```python
from build123d import *

# Parameters (mm, degrees)
F1_DEPTH = 72
F3_DEPTH = 30.001
F5_W     = 50
F5_H     = 6
F6_DEPTH = 72
F4_R     = 12
F7_DEPTH = 133.001
F8_DEPTH = 12.001


with BuildPart() as f1:
    # F0 (on Front) → F1 (new body)
    with BuildSketch(Plane.XZ):
        Polygon((-45.791163, 76.894684), (-81.791163, 76.894684), (-81.791163, 48.164527), (-69.791163, 48.164527), (-69.791163, 16.894684), (-81.791163, 16.894684), (-81.791163, -13.105316), (-9.791163, -13.105316), (63.208837, -13.105316), (63.208837, 16.894684), (-45.791163, 16.894684), align=None)
    extrude(amount=F1_DEPTH)

    # F2 (on face) → F3 (cut, through all)
    with BuildSketch(Plane.XY.offset(16.894684)):
        with BuildLine():
            Line((63.208837, -24), (13.208837, -24))
            ThreePointArc((13.208837, -24), (1.208837, -36), (13.208837, -48))
            Line((13.208837, -48), (63.208837, -48))
            Line((63.208837, -48), (63.208837, -24))
        make_face()
    extrude(amount=-F3_DEPTH, mode=Mode.SUBTRACT)

    # F5 (on face) → F6 (cut)
    with BuildSketch(Plane(origin=(-81.791163, 0, 0), x_dir=(0, -1, 0), z_dir=(-1, 0, 0))):
        with Locations((47, -10.105316)):
            Rectangle(F5_W, F5_H)
    extrude(amount=-F6_DEPTH, mode=Mode.SUBTRACT)

    # F4 (on face) → F7 (cut, through all)
    with BuildSketch(Plane(origin=(-69.791163, 0, 0), x_dir=(0, -1, 0), z_dir=(-1, 0, 0))):
        with Locations((36, 32.529606)):
            Circle(F4_R)
    extrude(amount=-F7_DEPTH, mode=Mode.SUBTRACT)

    # F4 (on face) → F8 (cut, through all)
    with BuildSketch(Plane(origin=(-69.791163, 0, 0), x_dir=(0, -1, 0), z_dir=(-1, 0, 0))):
        with Locations((36, 32.529606)):
            Circle(F4_R)
        with BuildLine():
            Line((61.603696, 16.894684), (10.396304, 16.894684))
            ThreePointArc((10.396304, 16.894684), (36, 2.529606), (61.603696, 16.894684))
        make_face()
        with BuildLine():
            Line((10.396304, 48.164527), (61.603696, 48.164527))
            ThreePointArc((61.603696, 48.164527), (36, 62.529606), (10.396304, 48.164527))
        make_face()
    extrude(amount=F8_DEPTH, mode=Mode.SUBTRACT)


solid = f1.part
```
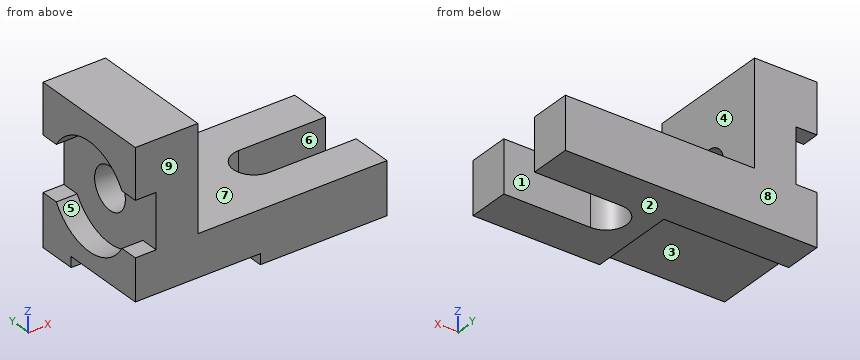
Part model, mm, in its own coordinate system. Face numbers are marked on the shaded views. A direction names the side the tool comes from. Round coordinates to 2 decimals unless told otherwise and drop trailing zeros. Order: outer loops, then holes, each group sorted by start corner. A loop starts at its lowest first (then second) coordinate and runs counter-clockwise, first axis right, second up. Notation, with made-up numbers: M 27,40.25 L 65,40.25 A30 cw 65,71.25 Z; hole C -11.5,-3 d4. An arc over 180 degrees is marked long. Put each result on its own line as item: value. Start each with the question number.
1. Slice it at D-D on y = -6.5. List the corners of the cut face in (x, z), then the cut area to 3 significant figures.
2. Drop flat-ended pins along their axis: pin 1 (3 mm diameter, centred on x = 6.5, z = -1.5, fed in from +Y); pin 2 (3 mm diameter, centred on x = -22, y = -42.5, fed in from -Z); pin 3 (21.5 mm diameter, centred on x = -3, y = -47, fed in from +Z); pin 4 (1.8 mm diameter, centred on x = -55.5, z = -11, fed in from -Y). Give the stop position or say it passes through.
3. Tool access for the marked faces 1, 2, 3, 4 and 5: list every direction of +Z, -Z, +X, -X, +Y, -Y with a clear straight run to the whole face (end or side of a thin tool).
4. Slice it at A-A on y = -36. List the corners of the cut face in (x, z).
5. Slice it at C-C on z = 40.5. List the corners of the cut face in (x, y).
6. Drill centre lines: probe 1 along Y at (x, z) = (15, -5.5); probe 2 along Z at (x, y) = (-59, -36); probe 3 along X at (y, z) = (-59.5, 63). Where is each one in solid material? Low to high. Write a range as [from, to].
7. Two-plate mould, pull along Y, no slides. Class the marked faces 6, 7, 8 and 9: +Y half, -Y half, draft (parallel to the pull), parting line (faces both ways), or undercut.
8. Slice it at B-B on x = 52.5. List the corners of the cut face in (y, z).
Findings:
1. outline: M -81.79,-13.11 L 63.21,-13.11 L 63.21,16.89 L -45.79,16.89 L -45.79,76.89 L -81.79,76.89 L -81.79,48.16 L -69.79,48.16 L -69.79,16.89 L -81.79,16.89 Z
1. area: 6,130 mm2
2. pin 1: y = 0
2. pin 2: z = -7.11
2. pin 3: z = 16.89
2. pin 4: y = -22
3. face 1: +Z, -Z, +X
3. face 2: -Z, +X, -X, +Y, -Y
3. face 3: -Z, -X, -Y
3. face 4: +Z, +X, +Y, -Y
3. face 5: -X
4. outline: M -81.79,-7.11 L -9.79,-7.11 L -9.79,-13.11 L 1.21,-13.11 L 1.21,16.89 L -45.79,16.89 L -45.79,20.53 L -69.79,20.53 L -69.79,2.53 L -81.79,2.53 Z; M -81.79,62.53 L -69.79,62.53 L -69.79,44.53 L -45.79,44.53 L -45.79,76.89 L -81.79,76.89 Z
5. outline: M -69.79,-72 L -45.79,-72 L -45.79,-44.97 L -69.79,-44.97 Z; M -69.79,-27.03 L -45.79,-27.03 L -45.79,0 L -69.79,0 Z
6. probe 1: [-72, -48], [-24, 0]
6. probe 2: [-7.11, 20.53], [44.53, 76.89]
6. probe 3: [-81.79, -45.79]
7. face 6: undercut
7. face 7: draft
7. face 8: +Y half
7. face 9: -Y half
8. outline: M -72,-13.11 L -48,-13.11 L -48,16.89 L -72,16.89 Z; M -24,-13.11 L 0,-13.11 L 0,16.89 L -24,16.89 Z
